from build123d import *

# Parameters (mm, degrees)
F0_R     = 3.5
F1_DEPTH = 7
F2_R     = 5.5
F3_DEPTH = 1
F5_R     = 0.49999
F4_R     = 5
F6_DEPTH = 7


# Not quite as in the source:
# - a fillet or chamfer is up to 0.001 mm smaller than in the source, because OpenCascade refuses the exact size


with BuildPart() as f1:
    # F0 (on Top) → F1 (new body)
    with BuildSketch(Plane.XY):
        Circle(F0_R)
    extrude(amount=F1_DEPTH)

    # F2 (on face) → F3 (join)
    with BuildSketch(Plane.XY.offset(7)):
        Circle(F2_R)
    extrude(amount=F3_DEPTH)

    # F5 (radius 0.5 in the source; OpenCascade refuses exactly that, so slightly less here)
    f5_edges = [f1.edges().sort_by_distance(p)[0] for p in [
        (-5.5, 0, 8),
        (-5.5, 0, 7),
    ]]
    fillet(f5_edges, radius=F5_R)

    # F4 (on face) → F6 (join)
    with BuildSketch(Plane.XY.offset(8)):
        Circle(F4_R)
    extrude(amount=F6_DEPTH)


solid = f1.part
Work out the finished part from the listing and answer in its coordinate system (mm). A direction names the side the tool comes from. Give positions to 0.01 mm unless a question says otherwise; leave off trailing zeros. Loops run counter-clockwise (first coordinate to the right, second up) from the corner with the lowest first, then second, coordinate; pieces in that order, holes last. Notation, with made-up numbers: (-10, -3) - (30, -3) arc R19 ccw to (30, 28) - close; hole circle Ø11 at (-21.75, 83). An arc over 180 degrees is marked (long way). Answer in a Markdown table with one row per item.
(1) Section C-C (z = 13.75) is taken. Give the vertices of the cut face in (x, y).
Results list:
| item | result |
|---|---|
| outline | circle Ø10 at (0, 0) |
(2) Flat-ended cylindrical pins translate along their axes: pin 1 Ø1 at (x, z) = (-1.5, 7.5) entering from -Y; pin 2 Ø4 at (y, z) = (-2, 4.5) entering from +X; pin 3 Ø5 at (y, z) = (0.5, 13) entering from +X. Find the tip coordinate at first contact, or state that the pin passes through.
Results list:
| item | result |
|---|---|
| pin 1 | stops at y = -5.41 |
| pin 2 | stops at x = 3.5 |
| pin 3 | stops at x = 5 |
(3) A tool of negligible diameter and unlimited length cuts with its end or side. For faces 1 (the face through (-1.08, -4.88, 11.45)), 2 (the face through (0, 0, 0)), 3 (the face through (2.2, -3.3, 7)), from which of +Z, -Z, +X, -X, +Y, -Y can it reach the whole face along a straight path? Write none if from no direction.
Results list:
| item | result |
|---|---|
| face 1 | +Z |
| face 2 | -Z, +X, -X, +Y, -Y |
| face 3 | -Z |
(4) Consider L1, parallel to Z at x = -0.5, y = 4.25; L2, parallel to Y at x = -2.5, z = 5.75; L3, parallel to X at y = -1.25, z = 10. Determine where each line is inside the solid, lowest interval first. Write a range as [from, to].
Results list:
| item | result |
|---|---|
| L1 | z = [7, 15] |
| L2 | y = [-2.45, 2.45] |
| L3 | x = [-4.84, 4.84] |
